```python
from build123d import *

# Parameters (mm, degrees)
BOSS_EXTRUDE1_DEPTH = 15
SKETCH2_R           = 7.067911596
BOSS_EXTRUDE2_DEPTH = 10


with BuildPart() as part:
    # Sketch1 → Boss-Extrude1 (new body)
    with BuildSketch(Plane(origin=(0, 0, 0), x_dir=(1, 0, 0), z_dir=(0, 1, 0))):
        Polygon((15.245454551, -7.948947663), (46.04976055, 6.529076156), (52.854431745, -7.948947663), (57.639851776, -5.699800249), (51.429912058, 9.057747365), (61.227828764, 13.662768217), (58.508060239, 19.44950976), (55.074851666, 19.44950976), (55.074851666, 47.693685978), (-35.770264484, 47.693685978), (-35.770264484, -7.948947663), align=None)
    extrude(amount=BOSS_EXTRUDE1_DEPTH)

    # Sketch2 → Boss-Extrude2 (add)
    with BuildSketch(Plane(origin=(55.074851666, 0, 0), x_dir=(0, 0, -1), z_dir=(1, 0, 0))):
        with Locations(Location((34.570742976, 7.378151278, 0), (0, 0, 180))):  # turned: the seam where the file's is
            Circle(SKETCH2_R)
    extrude(amount=BOSS_EXTRUDE2_DEPTH)


solid = part.part
```
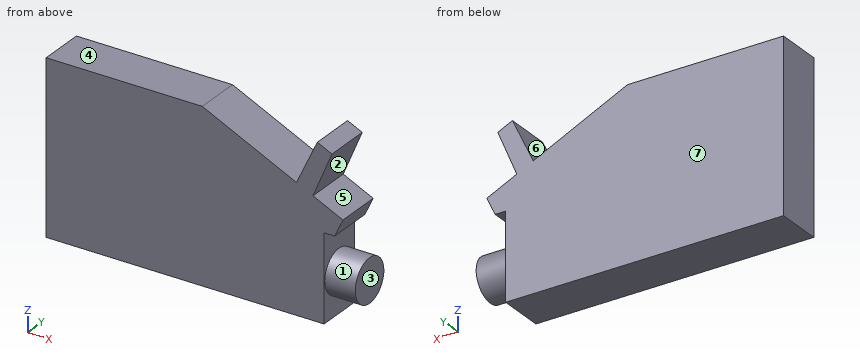
Here's how the part is built. I have some questions about the finished solid (model axes, mm). Face numbers are marked on the shaded views. A direction names the side the tool comes from. Give positions to 0.01 mm unless a question says otherwise; leave off trailing zeros. Order: outer loops, then holes, each group sorted by start corner. A loop starts at its lowest first (then second) coordinate and runs counter-clockwise, first axis right, second up. Notation, with made-up numbers: (11.5, 16) - (42.5, 16) arc R8 cw to (42.5, 25) - close; hole circle Ø5 at (82, 19.5). An arc over 180 degrees is marked (long way). Answer as a JSON object with one key per item and string values. Group by question number.
Item 1: If we mould it in two halves opening along Z, with no side actions, what happens to the marked faces 1, 2, 3 and 4? For each: pulls with the +Z half, pulls with the -Z half, needs draft (parallel to the pull), parting line crosses it, or undercut.
Item 2: Please list where these lines run through material, in increasing order: probe 1 along X at (y, z) = (8, -23); probe 2 along Z at (x, y) = (53, 2); probe 3 along Z at (x, y) = (27.5, 7.5).
Item 3: If we section it at C-C on y = 9: Please give me the cut outline in (x, z), and give its area (3 significant figures).
Item 4: If we section it at A-A on y = 1.5: Please give me the cut outline in (x, z), and give its area (3 significant figures).
Item 5: Which directions (+Z, -Z, +X, -X, +Y, -Y) give clear straight access to the entire face, cutting with the end or side of a thin tool? Please do the marked faces 5, 6 and 7.
Item 6: For P1, Ø1.5, axis at y = 8, z = -8, coming from the +X side; P2, Ø2.5, axis at x = 57, y = 7.5, coming from the -Z side, each with a flat end and sliding along its axis, tell me the tip position at first contact or that it passes through.
Item 7: If we section it at B-B on z = -30.5: Please give me the cut outline in (x, y).
Item 8: If we section it at D-D on z = -23.5: Please give me the cut outline in (x, y).
Result set:
{
 "1": {"face 1": "undercut", "face 2": "undercut", "face 3": "needs draft", "face 4": "pulls with the +Z half"},
 "2": {"probe 1": "-35.77 to 55.07", "probe 2": "-47.69 to -9.8, -5.33 to 7.88", "probe 3": "-47.69 to 2.19"},
 "3": {"outline": "(-35.77, -47.69) - (55.07, -47.69) - (55.07, -41.45) - (65.07, -41.45) - (65.07, -27.69) - (55.07, -27.69) - (55.07, -19.45) - (58.51, -19.45) - (61.23, -13.66) - (51.43, -9.06) - (57.64, 5.7) - (52.85, 7.95) - (46.05, -6.53) - (15.25, 7.95) - (-35.77, 7.95) - close", "area": "4,950 mm²"},
 "4": {"outline": "(-35.77, -47.69) - (55.07, -47.69) - (55.07, -38.5) - (65.07, -38.5) - (65.07, -30.65) - (55.07, -30.65) - (55.07, -19.45) - (58.51, -19.45) - (61.23, -13.66) - (51.43, -9.06) - (57.64, 5.7) - (52.85, 7.95) - (46.05, -6.53) - (15.25, 7.95) - (-35.77, 7.95) - close", "area": "4,890 mm²"},
 "5": {"face 5": "+X, +Y, -Y", "face 6": "+Z, +Y, -Y", "face 7": "+Z, -Z, +X, -X, +Y"},
 "6": {"P1": "x = 52.19", "P2": "z = -41.64"},
 "7": {"outline": "(-35.77, 0) - (55.07, 0) - (55.07, 1.6) - (65.07, 1.6) - (65.07, 13.16) - (55.07, 13.16) - (55.07, 15) - (-35.77, 15) - close"},
 "8": {"outline": "(-35.77, 0) - (55.07, 0) - (55.07, 15) - (-35.77, 15) - close"}
}
